Model file for the job. Use its own axes, mm. A direction names the side the tool comes from. Give positions to 0.01 mm unless a question says otherwise; leave off trailing zeros. Loops run counter-clockwise (first coordinate to the right, second up) from the corner with the lowest first, then second, coordinate; pieces in that order, holes last. Notation, with made-up numbers: M -23.5,44 L 16.5,44 A11 cw 16.5,62 Z; hole C 59.5,36 d5. An arc over 180 degrees is marked long. Use CSV: the item, a comma, the result in double quotes. Start each with the question number.
(1) Wall check: line 1 along Y through (x, z) = (-47.5, 2); line 2 along X through (y, z) = (-132.5, 20.5); line 3 along X through (y, z) = (-77.5, 11). Give the ranges that are in metal, low to high. Write a range as from..to.
(2) Slice it at A-A on z = 8. List the corners of the cut face in (x, y), and give its area (3 significant figures).
(3) Slice it at C-C on x = -17. List the corners of the cut face in (y, z).
(4) Tool access for faces 1 (the face through (-58, -43, 25.971)), 2 (the face through (-21, 0, 3)): list every direction of +Z, -Z, +X, -X, +Y, -Y with a clear straight run to the whole face (end or side of a thin tool).
(5) Slice it at B-B on y = -18. List the corners of the cut face in (x, z), and give its area (3 significant figures).
(6) Flat gauge pins, fed straight in: P1, Ø12, axis at y = -117, z = 8, coming from the +X side; P2, Ø12, axis at x = -50.5, y = -53, coming from the -Z side; P3, Ø8, axis at y = -112.5, z = -2.5, coming from the -X side. Where does each tip first touch, or does it go through?
```python
from build123d import *

# Parameters (mm, degrees)
SKETCH2_R           = 10
SKETCH2_R_2         = 1.275
BOSS_EXTRUDE1_DEPTH = 3
SKETCH3_R           = 1.275
BOSS_EXTRUDE2_DEPTH = 5
BOSS_EXTRUDE3_DEPTH = 5


with BuildPart() as part:
    # Sketch2 → Boss-Extrude1 (new body)
    with BuildSketch(Plane.XY):
        Circle(SKETCH2_R)
        with Locations((6.999985487, -0.014254341)):
            Circle(SKETCH2_R_2, mode=Mode.SUBTRACT)
        with Locations((-0.014254341, -6.999985487)):
            Circle(SKETCH2_R_2, mode=Mode.SUBTRACT)
        with Locations((-6.999985487, 0.014254341)):
            Circle(SKETCH2_R_2, mode=Mode.SUBTRACT)
        with Locations((0.014254341, 6.999985487)):
            Circle(SKETCH2_R_2, mode=Mode.SUBTRACT)
    extrude(amount=BOSS_EXTRUDE1_DEPTH)

    # Sketch3 → Boss-Extrude2 (add)
    with BuildSketch(Plane.XY.offset(3)):
        with BuildLine():
            Line((-0.02545418, -12.499974083), (-60.02532978, -12.377794019))
            Line((-60.02532978, -12.377794019), (-59.97442142, 12.622154148))
            Line((-59.97442142, 12.622154148), (0.02545418, 12.499974083))
            ThreePointArc((0.02545418, 12.499974083), (12.499974083, -0.02545418), (-0.02545418, -12.499974083))
        make_face()
        with Locations((6.999985487, -0.014254341)):
            Circle(SKETCH3_R, mode=Mode.SUBTRACT)
        with Locations((-0.014254341, -6.999985487)):
            Circle(SKETCH3_R, mode=Mode.SUBTRACT)
        with Locations((-6.999985487, 0.014254341)):
            Circle(SKETCH3_R, mode=Mode.SUBTRACT)
        with Locations((0.014254341, 6.999985487)):
            Circle(SKETCH3_R, mode=Mode.SUBTRACT)
    extrude(amount=-BOSS_EXTRUDE2_DEPTH)

    # Sketch4 → Boss-Extrude3 (add)
    with BuildSketch(Plane(origin=(-59.9998756, 0.122180064, 0), x_dir=(0.002036334, 0.999997927, 0), z_dir=(-0.999997927, 0.002036334, 0))):
        with BuildLine():
            Line((-62.942627893, -25.970573692), (-22.627671819, -25.970573692))
            Line((-22.627671819, -25.970573692), (12.5, -15.199288929))
            Line((12.5, -15.199288929), (12.5, -3))
            Line((12.5, -3), (-12.5, -3))
            Line((-12.5, -3), (-42.396291449, -12.167173681))
            Line((-42.396291449, -12.167173681), (-62.942627893, 2.349426308))
            add(Edge.make_bspline(
                [(-62.942627893, 2.349426308), (-87.492278411, -4.509248518), (-135.602543773, 45.42627104), (-139.208088658, -4.310573692)],
                knots=[0, 0, 0, 0, 1, 1, 1, 1], degree=3))
            Line((-139.208088658, -4.310573692), (-139.208088658, -19.310573692))
            add(Edge.make_bspline(
                [(-62.942627893, -25.970573692), (-87.492278411, -19.111898866), (-135.602543773, -69.047418424), (-139.208088658, -19.310573692)],
                knots=[0, 0, 0, 0, 1, 1, 1, 1], degree=3))
        make_face()
    extrude(amount=-BOSS_EXTRUDE3_DEPTH)


solid = part.part
```
Reply:
1,line 1,"y = -12.4..12.6"
1,line 2,"x = -60.27..-55.27"
1,line 3,"x = -60.16..-55.16"
2,outline,"M -60.28,-139.09 L -55.28,-139.1 L -55.1,-48.18 L -60.1,-48.17 Z; M -60.06,-28.68 L -55.06,-28.69 L -54.97,12.61 L -59.97,12.62 Z"
2,area,"661 mm^2"
3,outline,"M -12.47,-2 L 12.53,-2 L 12.53,3 L -12.47,3 Z"
4,face 1,"+Z, +X, -X, +Y"
4,face 2,"+Z, +X, +Y, -Y"
5,outline,"M -60.04,4.72 L -55.04,4.72 L -55.04,24.59 L -60.04,24.59 Z"
5,area,"99.3 mm^2"
6,P1,"stops at x = -55.23"
6,P2,"stops at z = 1.89"
6,P3,"stops at x = -60.24"
